Job drawing, mm, ordinate dimensions from the low corner. One solid piece. Give positions to 0.01 mm unless a question says otherwise; leave off trailing zeros. Loops run counter-clockwise (first coordinate to the right, second up) from the corner with the lowest first, then second, coordinate; pieces in that order, holes last. Notation, with made-up numbers: M 61.25,52 L 93.25,52 A14 cw 93.25,59 Z; hole C 86.5,31.5 d7. An arc over 180 degrees is marked long. Put each result on its own line as item: value.
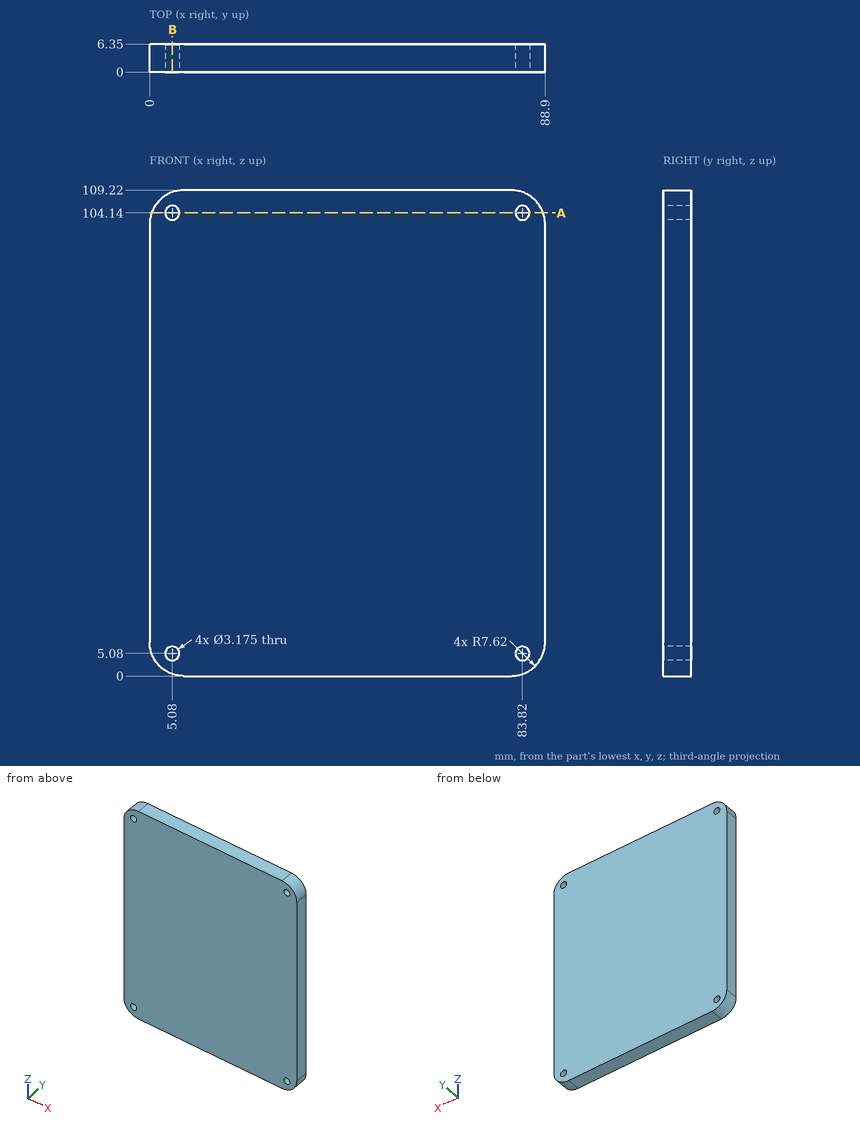
Q1. Slice it at B-B (x = 5.08). List the corners of the cut face in (y, z).
Here are the results:
outline: M 0,0.44 L 6.35,0.44 L 6.35,3.49 L 0,3.49 Z; M 0,6.67 L 6.35,6.67 L 6.35,102.55 L 0,102.55 Z; M 0,105.73 L 6.35,105.73 L 6.35,108.78 L 0,108.78 Z
Q2. Probe line 1 (Z direction, x = 5.08, y = 3.5); line 2 (X direction, y = 4.75, z = 5.08). List the from-to ranges inside material, lowest first. Write a range as from..to.
Here are the results:
line 1: 0.44..3.49, 6.67..102.55, 105.73..108.78
line 2: 0.44..3.49, 6.67..82.23, 85.41..88.46
Q3. Drop flat-ended pins along their axis: pin 1 Ø4 at (x, z) = (5.08, 104.14) entering from +Y; pin 2 Ø2.5 at (x, z) = (83.82, 5.08) entering from -Y. Give the stop position or say it passes through.
Here are the results:
pin 1: y = 6.35
pin 2: through
Q4. Slice it at A-A (z = 104.14). List the corners of the cut face in (x, y), and give its area (3 significant figures).
Here are the results:
outline: M 0.44,0 L 3.49,0 L 3.49,6.35 L 0.44,6.35 Z; M 6.67,0 L 82.23,0 L 82.23,6.35 L 6.67,6.35 Z; M 85.41,0 L 88.46,0 L 88.46,6.35 L 85.41,6.35 Z
area: 519 mm²
